Geometry check sheet. Reference: drawing and pictorial views, mm from the part's lowest x, y, z. Round coordinates to 2 decimals unless told otherwise and drop trailing zeros. Loops run counter-clockwise (first coordinate to the right, second up) from the corner with the lowest first, then second, coordinate; pieces in that order, holes last. Notation, with made-up numbers: (-0.5, -19.75) - (41.5, -19.75) arc R9 ccw to (41.5, -3.75) - close; hole circle Ø10 at (65, 73.5). An arc over 180 degrees is marked (long way). Answer as CSV lines item,"result". Start each with the question number.
1) Cross-section at B-B on x = 52.5. Record the boundary of the cut face in (y, z).
2) Cross-section at A-A on z = 20. Record the boundary of the cut face in (x, y) (3 decimals), and give its area (3 significant figures).
3) Thickness scan on line 1 along X through (y, z) = (2.75, 15) (3 decimals); line 2 along Z through (x, y) = (53, 1.35); line 3 along X through (y, z) = (1.95, 44). Record the ranges inside material, lowest first.
4) Cross-section at D-D on x = 38. Record the boundary of the cut face in (y, z), and give its area (3 significant figures).
5) Depth check by flat-ended pin: P1, Ø0.6, axis at x = 20, y = 1, coming from the +Z side; P2, Ø3, axis at x = 66, z = 24.5, coming from the -Y side; P3, Ø0.6, axis at y = 1, z = 24, coming from the -X side. Enter the tip coordinate at first touch or a pass-through.
6) Cross-section at C-C on y = 2.65. Record the boundary of the cut face in (x, z) (3 decimals), and give its area (3 significant figures).
7) Draft check along Z on the marked faces 1 and 2. Enter one of: released by +Z, released by -Z, zero draft, split by the parting line, or undercut.
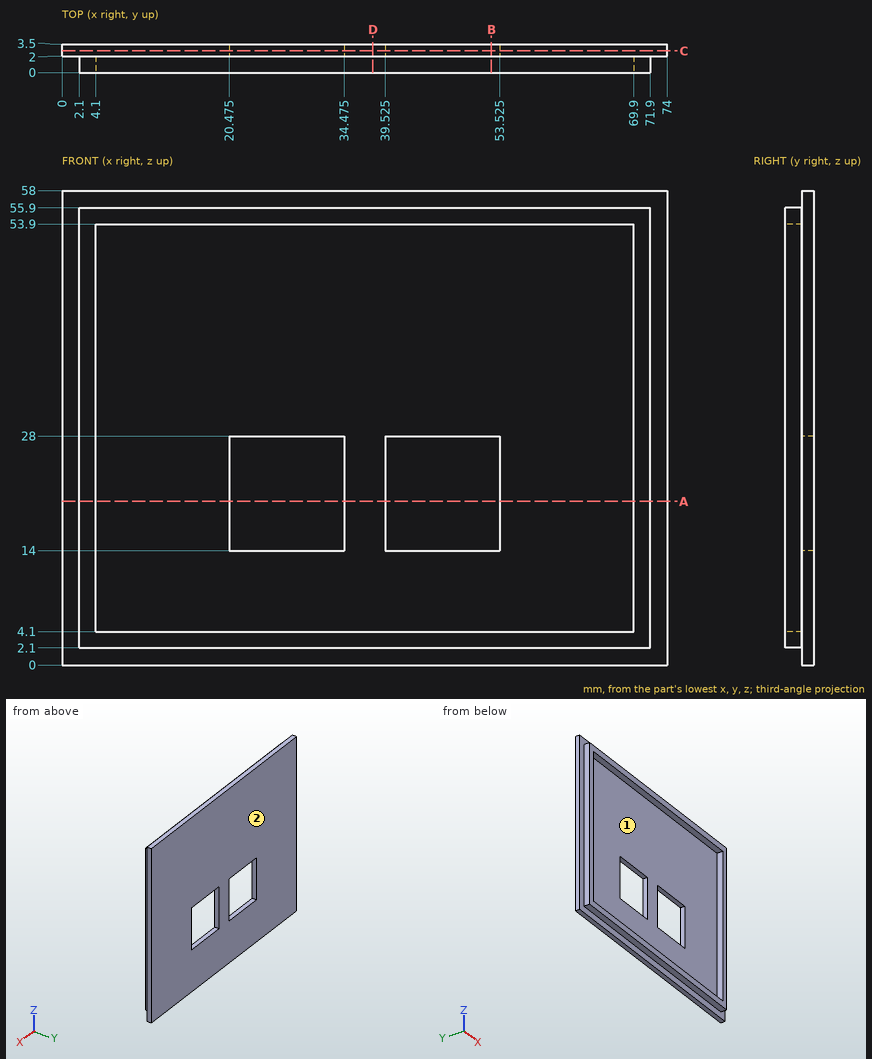
Answer block:
1,outline,"(0, 2.1) - (2, 2.1) - (2, 0) - (3.5, 0) - (3.5, 14) - (2, 14) - (2, 4.1) - (0, 4.1) - close; (0, 53.9) - (2, 53.9) - (2, 28) - (3.5, 28) - (3.5, 58) - (2, 58) - (2, 55.9) - (0, 55.9) - close"
2,outline,"(0, 2) - (2.1, 2) - (2.1, 0) - (4.1, 0) - (4.1, 2) - (20.475, 2) - (20.475, 3.5) - (0, 3.5) - close; (34.475, 2) - (39.525, 2) - (39.525, 3.5) - (34.475, 3.5) - close; (53.525, 2) - (69.9, 2) - (69.9, 0) - (71.9, 0) - (71.9, 2) - (74, 2) - (74, 3.5) - (53.525, 3.5) - close"
2,area,"77.0 mm^2"
3,line 1,"x = 0 to 20.475, 34.475 to 39.525, 53.525 to 74"
3,line 2,"z = 2.1 to 4.1, 53.9 to 55.9"
3,line 3,"x = 2.1 to 4.1, 69.9 to 71.9"
4,outline,"(0, 2.1) - (2, 2.1) - (2, 0) - (3.5, 0) - (3.5, 58) - (2, 58) - (2, 55.9) - (0, 55.9) - (0, 53.9) - (2, 53.9) - (2, 4.1) - (0, 4.1) - close"
4,area,"95.0 mm^2"
5,P1,"stops at z = 55.9"
5,P2,"stops at y = 2"
5,P3,"stops at x = 2.1"
6,outline,"(0, 0) - (74, 0) - (74, 58) - (0, 58) - close; hole (20.475, 14) - (34.475, 14) - (34.475, 28) - (20.475, 28) - close; hole (39.525, 14) - (53.525, 14) - (53.525, 28) - (39.525, 28) - close"
6,area,"3,900 mm^2"
7,face 1,"undercut"
7,face 2,"zero draft"
